Verification items for the finished model (mm, model axes). A direction names the side the tool comes from. Round coordinates to 2 decimals unless told otherwise and drop trailing zeros. Write each loop counter-clockwise with the first axis right and the second up, starting at its lowest first coordinate (ties: lowest second). Pieces come first, ordered by that corner, then holes. Notation, with made-up numbers: (0, 43) - (49, 43) arc R14 ccw to (49, 48) - close; hole circle Ø8 at (-21.75, 42.25). An arc over 180 degrees is marked (long way). Answer as a JSON object with one key per item and string values.
Autodesk Inventor part; units mm, degrees
ref_plane "YZ Plane" through (0, 0, 0) normal (1, 0, 0) x (0, 1, 0)
ref_plane "XZ Plane" through (0, 0, 0) normal (0, 1, 0) x (-1, 0, 0)
ref_plane "XY Plane" through (0, 0, 0) normal (0, 0, 1) x (1, 0, 0)
sketch "Sketch1" plane through (0, 0, 0) normal (0, 0, 1) x (1, 0, 0)
  line L0 (0, 0) -> (25.4, 0)
  line L1 (25.4, 0) -> (25.4, -50.8)
  line L2 (25.4, -50.8) -> (0, -50.8)
  line L3 (0, -50.8) -> (0, 0)
  line L4 (22.225, -3.175) -> (3.175, -3.175)
  line L5 (3.175, -3.175) -> (3.175, -47.625)
  line L6 (3.175, -47.625) -> (22.225, -47.625)
  line L7 (22.225, -47.625) -> (22.225, -3.175)
  dimension "d0" = 25.4
  dimension "d1" = 50.8
  dimension "d2" = 3.175
extrude "Extrusion1" add sketch "Sketch1" along normal blind 419.1
sketch "Sketch2" plane through (25.4, -50.8, 0) normal (1, 0, 0) x (0, 0, -1)
  circle A0 centre (-381, 25.4) radius 14.2875
  circle A1 centre (-38.1, 25.4) radius 14.2875
  line L0 (0, 50.8) -> (0, 0)
  line L1 (0, 0) -> (-419.1, 0)
  line L2 (-419.1, 0) -> (-419.1, 50.8)
  dimension "d5" = 38.1
  dimension "d6" = 25.4
  dimension "d7" = 28.575
  dimension "d8" = 25.4
  dimension "d9" = 38.1
  dimension "d10" = 28.575
  dimension "d13" = 342.9
extrude "Extrusion2" cut sketch "Sketch2" against normal blind 376.623
properties part number "DRL 6 Long"
1. Access from +Z, -Z, +X, -X, +Y, -Y to the whole of each face (thin tool, end or side, straight path). Record for faces 1 (the face through (1.61, -15.744, 391.53)), 2 (the face through (3.175, -25, 207)).
Completed:
{"face 1": "+X, -X", "face 2": "+Z, -Z"}
2. Mould release check, pull along Z, two halves, no side actions. Record for faces 3 (the face through (22.225, -26, 207)), 4 (the face through (1.61, -13.35, 30.42)), 5 (the face through (2, -27, 0)): released by +Z, released by -Z, zero draft, split by the parting line, or undercut.
Completed:
{"face 3": "zero draft", "face 4": "undercut", "face 5": "released by -Z"}
3. Material ranges on probe 1 along X at (y, z) = (-38.5, 111) (3 decimals); probe 2 along Y at (x, z) = (1.3, 38.1); probe 3 along Y at (x, z) = (5, 86) (3 decimals), recorded low to high. Write a range as from..to.
Completed:
{"probe 1": "x = 0..3.175, 22.225..25.4", "probe 2": "y = -50.8..-39.69, -11.11..0", "probe 3": "y = -50.8..-47.625, -3.175..0"}
4. Cross-section at C-C (z = 342.5). Record the boundary of the cut face in (x, y) (3 decimals), plus the area to 3 significant figures.
Completed:
{"outline": "(0, -50.8) - (25.4, -50.8) - (25.4, 0) - (0, 0) - close; hole (3.175, -47.625) - (22.225, -47.625) - (22.225, -3.175) - (3.175, -3.175) - close", "area": "444 mm^2"}
5. Cross-section at B-B (x = 13.75). Record the boundary of the cut face in (y, z) (3 decimals).
Completed:
{"outline": "(-50.8, 0) - (-47.625, 0) - (-47.625, 419.1) - (-50.8, 419.1) - close; (-3.175, 0) - (0, 0) - (0, 419.1) - (-3.175, 419.1) - close"}
6. Cross-section at A-A (y = -25.4). Record the boundary of the cut face in (x, z) (1 decimal).
Completed:
{"outline": "(0, 0) - (3.2, 0) - (3.2, 23.8) - (0, 23.8) - close; (0, 52.4) - (3.2, 52.4) - (3.2, 366.7) - (0, 366.7) - close; (0, 395.3) - (3.2, 395.3) - (3.2, 419.1) - (0, 419.1) - close; (22.2, 0) - (25.4, 0) - (25.4, 23.8) - (22.2, 23.8) - close; (22.2, 52.4) - (25.4, 52.4) - (25.4, 366.7) - (22.2, 366.7) - close; (22.2, 395.3) - (25.4, 395.3) - (25.4, 419.1) - (22.2, 419.1) - close"}
